Read the model definition and answer for the solid it produces. Units are mm, in the model's axes. A direction names the side the tool comes from. Coordinates: 2 decimals unless noted, no trailing zeros. Loops run counter-clockwise (first coordinate to the right, second up) from the corner with the lowest first, then second, coordinate; pieces in that order, holes last. Notation, with made-up numbers: M -10,-26 L 26,-26 A31 cw 26,11 Z; hole C 63.5,79.25 d11. An arc over 180 degrees is marked long. One line per item, written item: value. Start each with the question number.
1. The part is cut by section A-A (z = -11.5). Write down the section's boundary in (x, y).
2. The part is cut by section D-D (z = 36). Write down the section's boundary in (x, y), then the cut area to 3 significant figures.
3. The part is cut by section B-B (y = -123). Write down the section's boundary in (x, z), then the cut area to 3 significant figures.
4. Consider probe 1 along X at (y, z) = (-14.5, -23); probe 2 along X at (y, z) = (-137.5, 14); probe 3 along Y at (x, z) = (70.5, 19). Determine where each line is inside the solid, lowest interval first.
5. The part is cut by section C-C (x = -85). Write down the section's boundary in (y, z).
6. Flat-ended cylindrical pins translate along their axes: pin 1 (12 mm diameter, centred on x = 6.5, y = -74.5, fed in from -Z); pin 2 (12 mm diameter, centred on x = -158.5, z = 3, fed in from -Y); pin 3 (22 mm diameter, centred on x = 97.5, z = -9.5, fed in from -Y). Find the tip coordinate at first contact, or state that the pin passes through.
7. Determine the mould class of faces 6 (the face through (0, 124, -20)), 7 (the face through (-249.76, 10.99, 0.35)), 8 (the face through (-112, 168, -25)) for opening direction X: +X half, -X half, draft (parallel to the pull), parting line (faces both ways), or undercut.
8. For faces 1 (the face through (-1, 1, 50)), 2 (the face through (0, -122, 20)), 3 (the face through (0, -122, -20)), 4 (the face through (-1, -33, -50)), 5 (the face through (-20, 123, 0)), determine the directions among +Z, -Z, +X, -X, +Y, -Y from which every point of the face is accessible in a straight line to the end or side of a thin tool.
```python
from build123d import *

# Parameters (mm, degrees)
F0_R     = 250
F1_DEPTH = 25
F0_W     = 40
F0_H     = 40
F2_DEPTH = 50
F3_DEPTH = 20


with BuildPart() as f1:
    # F0 (on Top) → F1 (new body, symmetric)
    with BuildSketch(Plane.XY):
        Circle(F0_R)
        with BuildLine():
            ThreePointArc((20, 198.9974874213), (141.4213562373, 141.4213562373), (198.9974874213, 20))
            Line((198.9974874213, 20), (220.8077311516, 20))
            Line((220.8077311516, 20), (220.8077311516, -20))
            Line((220.8077311516, -20), (198.9974874213, -20))
            ThreePointArc((198.9974874213, -20), (141.4213562373, -141.4213562373), (20, -198.9974874213))
            Line((20, -198.9974874213), (20, -220.8077311516))
            Line((20, -220.8077311516), (-20, -220.8077311516))
            Line((-20, -220.8077311516), (-20, -198.9974874213))
            ThreePointArc((-20, -198.9974874213), (-141.4213562373, -141.4213562373), (-198.9974874213, -20))
            Line((-198.9974874213, -20), (-220.8077311516, -20))
            Line((-220.8077311516, -20), (-220.8077311516, 20))
            Line((-220.8077311516, 20), (-198.9974874213, 20))
            ThreePointArc((-198.9974874213, 20), (-141.4213562373, 141.4213562373), (-20, 198.9974874213))
            Line((-20, 198.9974874213), (-20, 220.8077311516))
            Line((-20, 220.8077311516), (20, 220.8077311516))
            Line((20, 220.8077311516), (20, 198.9974874213))
        make_face(mode=Mode.SUBTRACT)
        with BuildLine():
            ThreePointArc((-198.9974874213, -20), (-200, 0), (-198.9974874213, 20))
            Line((-198.9974874213, 20), (-220.8077311516, 20))
            Line((-220.8077311516, 20), (-220.8077311516, -20))
            Line((-220.8077311516, -20), (-198.9974874213, -20))
        make_face()
        with BuildLine():
            Line((20, -220.8077311516), (20, -198.9974874213))
            ThreePointArc((20, -198.9974874213), (0, -200), (-20, -198.9974874213))
            Line((-20, -198.9974874213), (-20, -220.8077311516))
            Line((-20, -220.8077311516), (20, -220.8077311516))
        make_face()
        with BuildLine():
            Line((220.8077311516, 20), (198.9974874213, 20))
            ThreePointArc((198.9974874213, 20), (199.7492146221, 10.012555012), (200, 0))
            ThreePointArc((200, 0), (199.7492146221, -10.012555012), (198.9974874213, -20))
            Line((198.9974874213, -20), (220.8077311516, -20))
            Line((220.8077311516, -20), (220.8077311516, 20))
        make_face()
        with BuildLine():
            ThreePointArc((-20, 198.9974874213), (0, 200), (20, 198.9974874213))
            Line((20, 198.9974874213), (20, 220.8077311516))
            Line((20, 220.8077311516), (-20, 220.8077311516))
            Line((-20, 220.8077311516), (-20, 198.9974874213))
        make_face()
    extrude(amount=F1_DEPTH, both=True)



with BuildPart() as f2:
    # F0 (on Top) → F2 (new body, symmetric)
    with BuildSketch(Plane.XY):
        with BuildLine():
            Line((20, 20), (45.8257569496, 20))
            ThreePointArc((45.8257569496, 20), (35.3553390593, 35.3553390593), (20, 45.8257569496))
            Line((20, 45.8257569496), (20, 20))
        make_face()
        with BuildLine():
            Line((20, 20), (20, 45.8257569496))
            ThreePointArc((20, 45.8257569496), (0, 50), (-20, 45.8257569496))
            Line((-20, 45.8257569496), (-20, 20))
            Line((-20, 20), (20, 20))
        make_face()
        with BuildLine():
            Line((-20, 20), (-20, 45.8257569496))
            ThreePointArc((-20, 45.8257569496), (-35.3553390593, 35.3553390593), (-45.8257569496, 20))
            Line((-45.8257569496, 20), (-20, 20))
        make_face()
        with BuildLine():
            Line((-20, -20), (-20, 20))
            Line((-20, 20), (-45.8257569496, 20))
            ThreePointArc((-45.8257569496, 20), (-50, 0), (-45.8257569496, -20))
            Line((-45.8257569496, -20), (-20, -20))
        make_face()
        with BuildLine():
            ThreePointArc((-45.8257569496, -20), (-35.3553390593, -35.3553390593), (-20, -45.8257569496))
            Line((-20, -45.8257569496), (-20, -20))
            Line((-20, -20), (-45.8257569496, -20))
        make_face()
        with BuildLine():
            ThreePointArc((-20, -45.8257569496), (0, -50), (20, -45.8257569496))
            Line((20, -45.8257569496), (20, -20))
            Line((20, -20), (-20, -20))
            Line((-20, -20), (-20, -45.8257569496))
        make_face()
        with BuildLine():
            ThreePointArc((20, -45.8257569496), (35.3553390593, -35.3553390593), (45.8257569496, -20))
            Line((45.8257569496, -20), (20, -20))
            Line((20, -20), (20, -45.8257569496))
        make_face()
        with BuildLine():
            ThreePointArc((45.8257569496, -20), (48.9453156465, -10.2154821845), (50, 0))
            ThreePointArc((50, 0), (48.9453156465, 10.2154821845), (45.8257569496, 20))
            Line((45.8257569496, 20), (20, 20))
            Line((20, 20), (20, -20))
            Line((20, -20), (45.8257569496, -20))
        make_face()
        with BuildLine():
            Line((-20, -20), (-20, 20))
            Line((-20, 20), (-45.8257569496, 20))
            ThreePointArc((-45.8257569496, 20), (-50, 0), (-45.8257569496, -20))
            Line((-45.8257569496, -20), (-20, -20))
        make_face()
        Rectangle(F0_W, F0_H)
        with BuildLine():
            ThreePointArc((-20, -45.8257569496), (0, -50), (20, -45.8257569496))
            Line((20, -45.8257569496), (20, -20))
            Line((20, -20), (-20, -20))
            Line((-20, -20), (-20, -45.8257569496))
        make_face()
        with BuildLine():
            ThreePointArc((45.8257569496, -20), (48.9453156465, -10.2154821845), (50, 0))
            ThreePointArc((50, 0), (48.9453156465, 10.2154821845), (45.8257569496, 20))
            Line((45.8257569496, 20), (20, 20))
            Line((20, 20), (20, -20))
            Line((20, -20), (45.8257569496, -20))
        make_face()
        with BuildLine():
            Line((20, 20), (20, 45.8257569496))
            ThreePointArc((20, 45.8257569496), (0, 50), (-20, 45.8257569496))
            Line((-20, 45.8257569496), (-20, 20))
            Line((-20, 20), (20, 20))
        make_face()
    extrude(amount=F2_DEPTH, both=True)


with BuildPart() as f1_1:
    add(f1.part)

    add(f2.part)  # F3 merges F2
    # F0 (on Top) → F3 (join, symmetric)
    with BuildSketch(Plane.XY):
        with BuildLine():
            ThreePointArc((-45.8257569496, -20), (-50, 0), (-45.8257569496, 20))
            Line((-45.8257569496, 20), (-198.9974874213, 20))
            ThreePointArc((-198.9974874213, 20), (-200, 0), (-198.9974874213, -20))
            Line((-198.9974874213, -20), (-45.8257569496, -20))
        make_face()
        with BuildLine():
            ThreePointArc((-20, 45.8257569496), (0, 50), (20, 45.8257569496))
            Line((20, 45.8257569496), (20, 198.9974874213))
            ThreePointArc((20, 198.9974874213), (0, 200), (-20, 198.9974874213))
            Line((-20, 198.9974874213), (-20, 45.8257569496))
        make_face()
        with BuildLine():
            ThreePointArc((45.8257569496, 20), (48.9453156465, 10.2154821845), (50, 0))
            ThreePointArc((50, 0), (48.9453156465, -10.2154821845), (45.8257569496, -20))
            Line((45.8257569496, -20), (198.9974874213, -20))
            ThreePointArc((198.9974874213, -20), (199.7492146221, -10.012555012), (200, 0))
            ThreePointArc((200, 0), (199.7492146221, 10.012555012), (198.9974874213, 20))
            Line((198.9974874213, 20), (45.8257569496, 20))
        make_face()
        with BuildLine():
            Line((20, -198.9974874213), (20, -45.8257569496))
            ThreePointArc((20, -45.8257569496), (0, -50), (-20, -45.8257569496))
            Line((-20, -45.8257569496), (-20, -198.9974874213))
            ThreePointArc((-20, -198.9974874213), (0, -200), (20, -198.9974874213))
        make_face()
    extrude(amount=F3_DEPTH, both=True)

    # F4 (on Front) → F5 (revolve, cut)
    with BuildSketch(Plane.XZ):
        Polygon((0, -50), (0, 0), (-24, 0), (-32, -50), align=None)
    revolve(axis=Axis((0, 0, -25), (0, 0, -1)), mode=Mode.SUBTRACT)


solid = f1_1.part
```
Answer block:
1. outline: C 0,0 d500; hole M -199,-20 A200 ccw -20,-199 L -20,-45.83 A50 cw -45.83,-20 Z; hole M -199,20 L -45.83,20 A50 cw -20,45.83 L -20,199 A200 ccw Z; hole C 0,0 d51.68; hole M 20,-199 A200 ccw 199,-20 L 45.83,-20 A50 cw 20,-45.83 Z; hole M 20,45.83 A50 cw 45.83,20 L 199,20 A200 ccw 20,199 Z
2. outline: C 0,0 d100
2. area: 7,850 mm2
3. outline: M -217.65,-25 L -157.71,-25 L -157.71,25 L -217.65,25 Z; M -20,-20 L 20,-20 L 20,20 L -20,20 Z; M 157.71,-25 L 217.65,-25 L 217.65,25 L 157.71,25 Z
3. area: 7,590 mm2
4. probe 1: x = -249.58 to -199.47, -47.85 to -23.58, 23.58 to 47.85, 199.47 to 249.58
4. probe 2: x = -208.79 to -145.24, -20 to 20, 145.24 to 208.79
4. probe 3: y = -239.85 to -187.16, -20 to 20, 187.16 to 239.85
5. outline: M -235.11,-25 L -181.04,-25 L -181.04,25 L -235.11,25 Z; M -20,-20 L 20,-20 L 20,20 L -20,20 Z; M 181.04,-25 L 235.11,-25 L 235.11,25 L 181.04,25 Z
6. pin 1: stops at z = -20
6. pin 2: stops at y = -198.1
6. pin 3: stops at y = -234.56
7. face 6: undercut
7. face 7: parting line
7. face 8: draft
8. face 1: +Z, +X, -X, +Y, -Y
8. face 2: +Z
8. face 3: -Z
8. face 4: -Z, +X, -X, +Y, -Y
8. face 5: +Z, -Z
